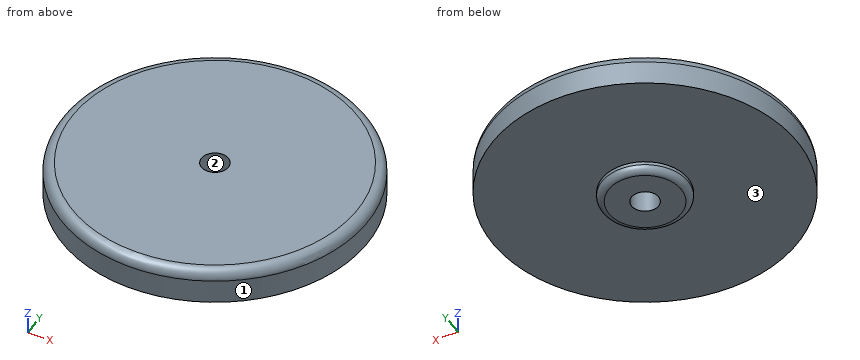
Autodesk Inventor part; units mm, degrees
ref_plane "YZ Plane" through (0, 0, 0) normal (1, 0, 0) x (0, 1, 0)
ref_plane "XZ Plane" through (0, 0, 0) normal (0, 1, 0) x (-1, 0, 0)
ref_plane "XY Plane" through (0, 0, 0) normal (0, 0, 1) x (1, 0, 0)
sketch "Sketch1" plane through (0, 0, 0) normal (0, 0, 1) x (1, 0, 0)
  circle A0 centre (0, 0) radius 3.925
  circle A1 centre (0, 0) radius 2
  dimension "d0" = 7.85
  dimension "d1" = 4
extrude "Extrusion1" add sketch "Sketch1" along normal blind 7
sketch "Sketch2" plane through (0, 0, 7) normal (0, 0, 1) x (1, 0, 0)
  circle A0 centre (0, 0) radius 22.5
  circle A1 centre (0, 0) radius 2
  dimension "d4" = 45
extrude "Extrusion2" add sketch "Sketch2" along normal blind 5.08
fillet "Fillet1" radius 1.5 1 edges at (-22.5, 0, 12.08)
sketch "Sketch4" plane through (0, 0, 7) normal (0, 0, -1) x (-1, 0, 0)
  circle A0 centre (0, 0) radius 3.925
  circle A1 centre (0, 0) radius 6.35
  dimension "d10" = 12.7
extrude "Extrusion4" add sketch "Sketch4" along normal blind 1.5
sketch "Sketch5" plane through (0, 0, 0) normal (0, 0, -1) x (-1, 0, 0)
  circle A0 centre (0, 0) radius 3.925
  circle A1 centre (0, 0) radius 2
fillet "Fillet2" radius 1 1 edges at (6.35, 0, 5.5)
extrude "Extrusion5" add sketch "Sketch5" along normal blind 1.5
sketch "Sketch6" plane through (0, 0, -1.5) normal (0, 0, -1) x (-1, 0, 0)
  circle A0 centre (0, 0) radius 3.925
  circle A1 centre (0, 0) radius 2
extrude "Extrusion6" cut sketch "Sketch6" against normal up to surface (7 mm away)
properties part number "wheel_mrrover2"
Input: part model. Units: mm. Frame: model coordinates. Face numbers are marked on the shaded views. Give positions to 0.01 mm unless a question says otherwise; leave off trailing zeros. Write each loop counter-clockwise with the first axis right and the second up, starting at its lowest first coordinate (ties: lowest second). Pieces come first, ordered by that corner, then holes.
Q1. Pull-direction query (Y, two-part tool) for the marked faces 1, 2 and 3; classes: pulls with the +Y half, pulls with the -Y half, needs draft (parallel to the pull), parting line crosses it, or undercut.
Q2. Section A-A, the plane y = 0. Output: boundary loops of the cut face in (x, z).
Q3. Material intervals for probe 1 along Y at (x, z) = (0, 7.5); probe 2 along Z at (x, y) = (-14, 2.5); probe 3 along X at (y, z) = (0.5, 10), sorted ascending.
Q4. First-contact query: P1, Ø2, axis at x = 14.5, z = 10, coming from the -Y side; P2, Ø1, axis at x = -12, y = 14.5, coming from the -Z side; P3, Ø3, axis at y = -14, z = 8, coming from the -X side; P4, Ø3.5, axis at x = 0, y = 0, coming from the +Z side. Flat tips, straight axial feed; report the tip coordinate or a pass-through.
Filled in:
1. face 1: parting line crosses it
1. face 2: undercut
1. face 3: needs draft
2. outline: (-22.5, 7) - (-6.35, 7) - (-6.35, 6.5) arc R1 ccw to (-5.35, 5.5) - (-2, 5.5) - (-2, 12.08) - (-21, 12.08) arc R1.5 ccw to (-22.5, 10.58) - close; (2, 5.5) - (5.35, 5.5) arc R1 ccw to (6.35, 6.5) - (6.35, 7) - (22.5, 7) - (22.5, 10.58) arc R1.5 ccw to (21, 12.08) - (2, 12.08) - close
3. probe 1: y = -22.5 to -2, 2 to 22.5
3. probe 2: z = 7 to 12.08
3. probe 3: x = -22.49 to -1.94, 1.94 to 22.49
4. P1: stops at y = -18
4. P2: stops at z = 7
4. P3: stops at x = -18.71
4. P4: passes through
